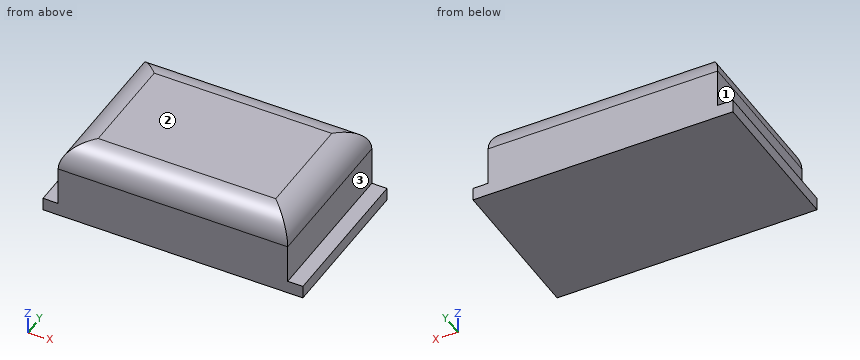
Autodesk Fusion 360 part; units mm, degrees
sketch "Sketch1" plane through (0, 0, 0) normal (0, 0, 1) x (1, 0, 0)
  line L0 (-30, 20) -> (-12.335, 20)
  line L1 (-12.335, 20) -> (-12.335, 8)
  line L2 (-12.335, 8) -> (-30, 8)
  line L3 (-30, 8) -> (-30, 20)
  dimension "d1" = 17.665
  dimension "d2" = 12
extrude "Extrude1" add sketch "Sketch1" along normal blind 6
fillet "Fillet1" radius 2 4 edges at (-21.1675, 20, 6) (-12.335, 14, 6) (-30, 14, 6) (-21.1675, 8, 6)
sketch "Sketch2" plane through (0, 0, 0) normal (0, 0, -1) x (-1, 0, 0)
  line L0 (12.335, 8) -> (30, 8)
  line L1 (30, 8) -> (30, 20)
  line L2 (30, 20) -> (12.335, 20)
  line L3 (12.335, 20) -> (12.335, 8)
  line L4 (11.1675, 20) -> (31.1675, 20)
  line L5 (11.1675, 8) -> (31.1675, 8)
  line L6 (31.1675, 20) -> (31.1675, 8)
  line L7 (11.1675, 8) -> (11.1675, 20)
  point P0 (21.1675, 20)
  point P1 (21.1675, 8)
  dimension "d7" = 20
extrude "Extrude2" add sketch "Sketch2" against normal blind 1 contours L3 L4 L5 L7 | L1 L4 L5 L6
Input: part model. Units: mm. Frame: model coordinates. Face numbers are marked on the shaded views. A direction names the side the tool comes from. Give positions to 0.01 mm unless a question says otherwise; leave off trailing zeros. Loops run counter-clockwise (first coordinate to the right, second up) from the corner with the lowest first, then second, coordinate; pieces in that order, holes last. Notation, with made-up numbers: (14.25, -18) -> (73.25, -18) arc R21 cw to (73.25, 4) -> close; hole circle Ø1 at (76.25, -11). An arc over 180 degrees is marked (long way). Answer as a JSON object with one key per item and string values. Group by question number.
Item 1: Pin query (flat end, axial travel): P1, Ø3.5, axis at y = 13, z = 3, coming from the -X side; P2, Ø0.6, axis at x = -30.5, y = 11.5, coming from the +Z side; P3, Ø1.5, axis at y = 12, z = 2.5, coming from the +X side (3 decimals). Return the tip coordinate at first contact, or that it passes through.
Item 2: Cut plane D-D, the plane x = -29.75. Return the cut outline in (y, z).
Item 3: Reachability of the marked faces 1, 2 and 3 from +Z, -Z, +X, -X, +Y, -Y: full face, straight path, thin tool, end or side. Return the list, or none.
Item 4: Cut plane A-A, the plane y = 15. Return the cut outline in (x, z) (1 decimal), and give its area (3 significant figures).
Item 5: Cut plane B-B, the plane z = 2.7. Return the cut outline in (x, y) (3 decimals).
Item 6: Line query: probe 1 along X at (y, z) = (12.25, 2.65) (3 decimals); probe 2 along Z at (x, y) = (-11.75, 10.25); probe 3 along Z at (x, y) = (-29, 10.75). Output: solid intervals per line, ascending.
Item 7: Cut plane C-C, the plane x = -19. Return the cut outline in (y, z).
Checks:
{
 "1": {"P1": "stops at x = -30", "P2": "stops at z = 1", "P3": "stops at x = -12.335"},
 "2": {"outline": "(8, 0) -> (20, 0) -> (20, 4) arc R2 ccw to (19.75, 4.97) -> (8.25, 4.97) arc R2 ccw to (8, 4) -> close"},
 "3": {"face 1": "+Z, -X, +Y, -Y", "face 2": "+Z, +X, -X, +Y, -Y", "face 3": "+Z, +X, +Y, -Y"},
 "4": {"outline": "(-31.2, 0) -> (-11.2, 0) -> (-11.2, 1) -> (-12.3, 1) -> (-12.3, 4) arc R2 ccw to (-14.3, 6) -> (-28, 6) arc R2 ccw to (-30, 4) -> (-30, 1) -> (-31.2, 1) -> close", "area": "107 mm²"},
 "5": {"outline": "(-30, 8) -> (-12.335, 8) -> (-12.335, 20) -> (-30, 20) -> close"},
 "6": {"probe 1": "x = -30 to -12.335", "probe 2": "z = 0 to 1", "probe 3": "z = 0 to 5.73"},
 "7": {"outline": "(8, 0) -> (20, 0) -> (20, 4) arc R2 ccw to (18, 6) -> (10, 6) arc R2 ccw to (8, 4) -> close"}
}
